For this review, take the finished solid that the model builds, in its own axes (mm). A direction names the side the tool comes from. Give positions to 0.01 mm unless a question says otherwise; leave off trailing zeros. Write each loop counter-clockwise with the first axis right and the second up, starting at its lowest first coordinate (ties: lowest second). Pieces come first, ordered by that corner, then holes.
Q1. We need section C-C (x = 9). Write out the cut boundary in (y, z), then the cut area to 3 significant figures.
Q2. Mouldability with a two-part tool opening along Z and no side actions: class faces 6 (the cylindrical face through (-0.29, 2.46, 2.23)), 7 (the flat face through (5, 0, 0)), 8 (the cylindrical face through (9.13, 12.23, -14.41)), 9 (the cylindrical face through (23.463, 3.724, 9.728)) as released by +Z, released by -Z, zero draft, split by the parting line, or undercut.
Q3. We need section A-A (y = 8). Write out the cut boundary in (x, z).
Q4. Machinability: for faces 1 (the flat face through (20, 29, -7)), 2 (the cylindrical face through (3.815, 10.445, -1.201)), 3 (the flat face through (10.9, 30.7, -4.75)), 4 (the flat face through (5, 29, -7)), 5 (the flat face through (14.1, 30.7, 10)), which of the approach directions +Z, -Z, +X, -X, +Y, -Y give a long, thin tool a straight path to every point of the face, cutting with its end or side? Answer none if there is none.
Q5. We need section B-B (z = -11). Write out the cut boundary in (x, y).
Q6. Insertion check: P1, Ø1, axis at y = 8, z = 16.5, coming from the -X side; P2, Ø3, axis at y = 21, z = -8, coming from the -X side; P3, Ø4, axis at x = -0.5, z = -1, coming from the +Y side; P4, Ø2.5, axis at x = 12.5, y = 32.5, coming from the -Z side. Each pin has a flat end and moves straight along its axis. Give the tip position at first contact, or say it passes through.
Q7. For line 1 (Z direction, x = 0, y = 3.8); line 2 (Z direction, x = 16.5, y = 25.5); line 3 (Y direction, x = 1, z = -3), list the stretches that pass through material, from the lowest coordinate up.
Q8. We need section D-D (z = 7). Write out the cut boundary in (x, y).
```python
from build123d import *

# Parameters (mm, degrees)
SKETCH1_R               = 25.4
BASE_DEPTH              = 25
SKETCH3_OUTSIDE_W       = 68.014
SKETCH3_OUTSIDE_H       = 42.214
CUT_EXTRUDE1_DEPTH      = 26.4
CUT_EXTRUDE1_DEPTH_BACK = 26.4
SKETCH4_OUTSIDE_W       = 68.014
SKETCH4_OUTSIDE_H       = 42.214
CUT_EXTRUDE2_DEPTH      = 26.4000001
CUT_EXTRUDE2_DEPTH_BACK = 26.4000001
SKETCH5_R               = 2.25
CUT_EXTRUDE3_DEPTH      = 26.0000001
SKETCH6_R               = 4
CUT_EXTRUDE4_DEPTH      = 20
SKETCH7_W               = 15
SKETCH7_H               = 20
ARM_BASE_DEPTH          = 15
SKETCH8_R               = 2.25
ARM_HOLE_DEPTH          = 36.4000001
SKETCH9_W               = 9.5
SKETCH9_H               = 15
CUT_EXTRUDE7_DEPTH      = 46.4000001


with BuildPart() as part:
    # Sketch1 → base (new body)
    with BuildSketch(Plane(origin=(0, 0, 0), x_dir=(1, 0, 0), z_dir=(0, 1, 0))):
        Circle(SKETCH1_R)
    extrude(amount=BASE_DEPTH)

    # Sketch3 outside → Cut-Extrude1 (cut, two sides)
    with BuildSketch(Plane.XY) as cut_extrude1_sk:
        with Locations((0, 12.5)):
            Rectangle(SKETCH3_OUTSIDE_W, SKETCH3_OUTSIDE_H)
        with BuildLine():
            Line((5, 25), (20, 25))
            ThreePointArc((20, 25), (21.373745827, 14.641911373), (25.4, 5))
            Line((25.4, 5), (25.4, 0))
            Line((25.4, 0), (-25.4, 0))
            Line((-25.4, 0), (-25.4, 5))
            Line((-25.4, 5), (-15, 5))
            ThreePointArc((-15, 5), (-0.857864376, 10.857864376), (5, 25))
        make_face(mode=Mode.SUBTRACT)
    extrude(amount=CUT_EXTRUDE1_DEPTH, mode=Mode.SUBTRACT)
    extrude(cut_extrude1_sk.sketch, amount=-CUT_EXTRUDE1_DEPTH_BACK, mode=Mode.SUBTRACT)

    # Sketch4 outside → Cut-Extrude2 (cut, two sides)
    with BuildSketch(Plane(origin=(0, 0, 0), x_dir=(0, 0, -1), z_dir=(1, 0, 0))) as cut_extrude2_sk:
        with Locations((0, 12.5)):
            Rectangle(SKETCH4_OUTSIDE_W, SKETCH4_OUTSIDE_H)
        with BuildLine():
            Line((-25.4, 5), (-25.4, 0))
            Line((-25.4, 0), (25.4, 0))
            Line((25.4, 0), (25.4, 5))
            ThreePointArc((25.4, 5), (14.296085426, 12.378985778), (10, 25))
            Line((10, 25), (-10, 25))
            ThreePointArc((-10, 25), (-14.296085426, 12.378985778), (-25.4, 5))
        make_face(mode=Mode.SUBTRACT)
    extrude(amount=CUT_EXTRUDE2_DEPTH, mode=Mode.SUBTRACT)
    extrude(cut_extrude2_sk.sketch, amount=-CUT_EXTRUDE2_DEPTH_BACK, mode=Mode.SUBTRACT)

    # Sketch5 → Cut-Extrude3 (cut, through all)
    with BuildSketch(Plane.XZ):
        Circle(SKETCH5_R)
    extrude(amount=-CUT_EXTRUDE3_DEPTH, mode=Mode.SUBTRACT)

    # Sketch6 → Cut-Extrude4 (cut)
    with BuildSketch(Plane(origin=(0, 25, 0), x_dir=(1, 0, 0), z_dir=(0, 1, 0))):
        Circle(SKETCH6_R)
    extrude(amount=-CUT_EXTRUDE4_DEPTH, mode=Mode.SUBTRACT)

    # Sketch7 → arm base (add)
    with BuildSketch(Plane(origin=(0, 25, 0), x_dir=(1, 0, 0), z_dir=(0, 1, 0))):
        with Locations((12.5, 0)):
            Rectangle(SKETCH7_W, SKETCH7_H)
    extrude(amount=ARM_BASE_DEPTH)

    # Sketch8 → arm hole (cut, through all)
    with BuildSketch(Plane(origin=(0, 0, -10), x_dir=(-1, 0, 0), z_dir=(0, 0, -1))):
        with BuildLine():
            ThreePointArc((-12.5, 40), (-7.196699141, 37.803300859), (-5, 32.5))
            Line((-5, 32.5), (-5, 40))
            Line((-5, 40), (-12.5, 40))
        make_face()
        with BuildLine():
            ThreePointArc((-20, 32.5), (-17.803300859, 37.803300859), (-12.5, 40))
            Line((-12.5, 40), (-20, 40))
            Line((-20, 40), (-20, 32.5))
        make_face()
        with Locations((-12.5, 32.5)):
            Circle(SKETCH8_R)
    extrude(amount=-ARM_HOLE_DEPTH, mode=Mode.SUBTRACT)

    # Sketch9 → Cut-Extrude7 (cut, through all)
    with BuildSketch(Plane(origin=(20, 0, 0), x_dir=(0, 0, -1), z_dir=(1, 0, 0))):
        with Locations((0, 32.5)):
            Rectangle(SKETCH9_W, SKETCH9_H)
    extrude(amount=-CUT_EXTRUDE7_DEPTH, mode=Mode.SUBTRACT)


solid = part.part
```
Computed:
1. outline: (0, -23.75) - (5.51, -23.75) arc R20.69 cw to (25, -10) - (39.13, -10) - (39.13, -4.75) - (25, -4.75) - (25, 4.75) - (39.13, 4.75) - (39.13, 10) - (25, 10) arc R20.69 cw to (5.51, 23.75) - (0, 23.75) - close
1. area: 945 mm2
2. face 6: undercut
2. face 7: zero draft
2. face 8: released by -Z
2. face 9: split by the parting line
3. outline: (-4.46, -18.9) - (16.97, -18.9) arc R25.4 ccw to (23.82, -8.82) - (23.82, 8.82) arc R25.4 ccw to (16.97, 18.9) - (-4.46, 18.9) - close; hole circle Ø8 at (0, 0)
4. face 1: +Z, -Z, +X, +Y
4. face 2: +Y
4. face 3: +X, -X, +Y
4. face 4: +Z, -Z, -X, +Y
4. face 5: +Z, +X, -X, +Y
5. outline: (-22.89, 0) - (22.89, 0) - (22.89, 10.11) arc R39.74 cw to (20.51, 18.65) - (3.96, 18.65) arc R20 cw to (-15, 5) - (-22.89, 5) - close
6. P1: stops at x = -5.32
6. P2: stops at x = 4.23
6. P3: stops at y = 5
6. P4: passes through
7. line 1: z = -25.4 to -2.25, 2.25 to 25.4
7. line 2: z = -10 to -4.75, 4.75 to 10
7. line 3: y = 0 to 5
8. outline: (-24.42, 0) - (24.42, 0) - (24.42, 6.79) arc R39.74 cw to (20, 25) - (20, 32.5) arc R7.5 ccw to (5, 32.5) - (5, 25) arc R20 cw to (-15, 5) - (-24.42, 5) - close; hole circle Ø4.5 at (12.5, 32.5)
